The listing builds one solid part. Answer for the finished solid, in the listing's coordinates (mm). Coordinates: 2 decimals unless noted, no trailing zeros. Loops run counter-clockwise (first coordinate to the right, second up) from the corner with the lowest first, then second, coordinate; pieces in that order, holes last. Notation, with made-up numbers: M -9,20.25 L 1,20.25 A37 ccw 1,59.25 Z; hole C -7.75,53.5 d11. An arc over 180 degrees is marked long. Return JSON: item names as keys, results as strings. Group by question number.
1. Given P1, Ø1, axis at y = 27.5, z = 38, coming from the +X side; P2, Ø0.9, axis at y = 129, z = 35, coming from the +X side; P3, Ø2.5, axis at x = 62.5, z = 37, coming from the +Y side; P4, Ø1.2, axis at y = 92, z = 35.5, coming from the -X side, each flat-ended and moving along its own axis, determine where each tip first touches the part or whether it passes through.
2. Straight lines are drawn through the part: L1, parallel to Y at x = 58, z = 35.75; L2, parallel to Y at x = -1.5, z = 36.5. For each, find the intervals that lie inside material, in ascending order. Write a range as from..to.
3. Section A-A (x = 26) is taken. Write down the section's boundary in (y, z).
4. Section B-B (y = 211.5) is taken. Write down the section's boundary in (x, z).
5. Section C-C (z = 38.5) is taken. Write down the section's boundary in (x, y).
```python
from build123d import *

# Parameters (mm, degrees)
PAD008_DEPTH    = 0.25
SKETCH021_W     = 101.318497
SKETCH021_H     = 15.372729
POCKET001_DEPTH = 41.578934
SKETCH020_W     = 85.083054
SKETCH020_H     = 0.25
PAD009_DEPTH    = 10


with BuildPart() as part:
    # AdditivePipe005: sweep along a path in Sketch016
    with BuildLine(Plane.XY) as additivepipe005_path:
        Line((-18.15, 227), (-18.15, -17))
        ThreePointArc((-18.15, -17), (-17.8131727984, -17.8131727984), (-17, -18.15))
        Line((-17, -18.15), (59, -18.15))
        ThreePointArc((59, -18.15), (59.8131727984, -17.8131727984), (60.15, -17))
        Line((60.15, -17), (60.15, 227))
        ThreePointArc((60.15, 227), (59.8131727984, 227.8131727984), (59, 228.15))
        Line((59, 228.15), (-17, 228.15))
        ThreePointArc((-17, 228.15), (-17.8131727984, 227.8131727984), (-18.15, 227))
    # Sketch015 → AdditivePipe005 (sweep)
    with BuildSketch(Plane.XZ):
        Polygon((-18.15, 36.6), (-18.9, 35.85), (-18.9, 35.1), (-18.15, 35.1), (-18.15, 34.85), (-19.15, 34.85), (-19.15, 35.9535533906), (-18.15, 36.9535533906), align=None)
    sweep(path=additivepipe005_path.line)

    # Sketch019 → Pad008 (new body)
    with BuildSketch(Plane.XZ.offset(17)):
        Polygon((-18.15, 36.9535533906), (-18.15, 41.577934), (-21.541527, 41.577934), (-21.541527, 34.85), (-19.15, 34.85), (-19.15, 35.9535533906), align=None)
        Polygon((60.15, 36.9535533906), (60.15, 41.577934), (63.541527, 41.577934), (63.541527, 34.85), (61.15, 34.85), (61.15, 35.9535533906), align=None)
    extrude(amount=-PAD008_DEPTH)

    # Sketch021 → Pocket001 (cut, through all)
    with BuildSketch(Plane.XY):
        with Locations((14.6124585, -24.6863645)):
            Rectangle(SKETCH021_W, SKETCH021_H)
    extrude(amount=POCKET001_DEPTH, mode=Mode.SUBTRACT)

    # Sketch020 (on Face13 of Pad008) → Pad009 (join)
    with BuildSketch(Plane.XZ.offset(17)):
        with Locations((21, 34.975)):
            Rectangle(SKETCH020_W, SKETCH020_H)
    extrude(amount=PAD009_DEPTH)


solid = part.part
```
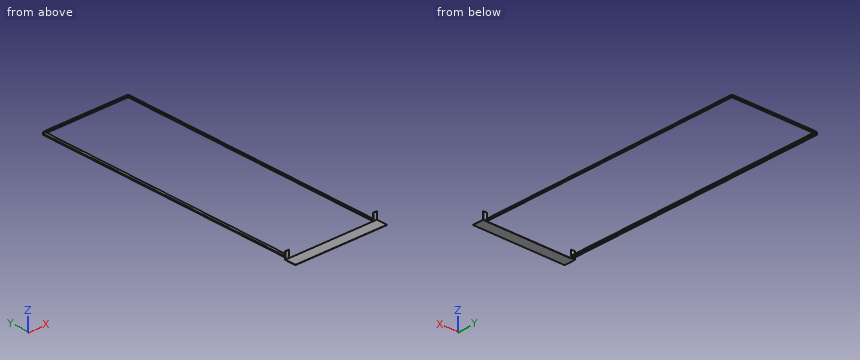
Worked out:
{
 "1": {"P1": "through", "P2": "x = 61.15", "P3": "y = -16.75", "P4": "x = -19.15"},
 "2": {"L1": "228.9..229.15", "L2": "228.25..228.6"},
 "3": {"outline": "M -27,34.85 L -17,34.85 L -17,35.1 L -27,35.1 Z; M 228.15,34.85 L 229.15,34.85 L 229.15,35.95 L 228.15,36.95 L 228.15,36.6 L 228.9,35.85 L 228.9,35.1 L 228.15,35.1 Z"},
 "4": {"outline": "M -19.15,34.85 L -18.15,34.85 L -18.15,35.1 L -18.9,35.1 L -18.9,35.85 L -18.15,36.6 L -18.15,36.95 L -19.15,35.95 Z; M 60.15,34.85 L 61.15,34.85 L 61.15,35.95 L 60.15,36.95 L 60.15,36.6 L 60.9,35.85 L 60.9,35.1 L 60.15,35.1 Z"},
 "5": {"outline": "M -21.54,-17 L -18.15,-17 L -18.15,-16.75 L -21.54,-16.75 Z; M 60.15,-17 L 63.54,-17 L 63.54,-16.75 L 60.15,-16.75 Z"}
}
